For this review, take the finished solid that the model builds, in its own axes (mm). A direction names the side the tool comes from. Coordinates: 2 decimals unless noted, no trailing zeros. Loops run counter-clockwise (first coordinate to the right, second up) from the corner with the lowest first, then second, coordinate; pieces in that order, holes last. Notation, with made-up numbers: M 72.5,68.5 L 103.5,68.5 A12 cw 103.5,73.5 Z; hole C 65,-14.5 d6. An arc over 180 degrees is marked long. Answer as a JSON object with one key per item and string values. Group by question number.
Item 1: Add section A-A (x = -9.5). State the section outline as (y, z) points, then the cut area to 3 significant figures.
Item 2: Insertion check: pin 1 (1 mm diameter, centred on x = 9, z = -35, fed in from +Y); pin 2 (3 mm diameter, centred on x = 39, z = -39, fed in from -Y); pin 3 (1 mm diameter, centred on x = 6, y = 0.5, fed in from -Z); pin 4 (1.6 mm diameter, centred on x = 43.5, y = 3, fed in from +Z). Each pin has a flat end and moves straight along its axis. Give the tip position at first contact, or say it passes through.
Item 3: Tool access review of faces 4 (the face through (42, 3, -32.785)), 5 (the face through (-42, 3, 32.785)), 6 (the face through (33.607, 1.014, -44.132)), 7 (the face through (0, 1, 40.021)): name each direction out of +Z, -Z, +X, -X, +Y, -Y from which nothing blocks a thin tool from reaching the whole face with its end or side.
Item 4: Wall thickness on L1, parallel to X at y = 1, z = -39; L2, parallel to Z at x = 11, y = 0.2; L3, parallel to X at y = 3.45, z = -20: over which ranges is each line inside the solid? List them lowest first. Write a range as from..to.
Item 5: Mouldability with a two-part tool opening along Z and no side actions: class faces 1 (the face through (42, 3, 32.785)), 2 (the face through (37.418, 0.986, -41.063)), 3 (the face through (-42, 3, -32.785)) as +Z half, -Z half, draft (parallel to the pull), parting line (faces both ways), or undercut.
Item 6: Add section D-D (z = 39). State the section outline as (x, y) points.
Item 7: Add section C-C (y = 2.95). State the section outline as (x, z) points, then the cut area to 3 significant figures.
Item 8: Add section B-B (z = -24). State the section outline as (x, y) points.
from build123d import *

# Parameters (mm, degrees)
SKETCH_1_W          = 90.03018306390481
SKETCH_1_H          = 89.97022234109225
SKETCH_1_R          = 2.599999999999996
SKETCH_1_W_2        = 65.97077516555349
SKETCH_1_H_2        = 66.02977765890743
EXTRUDE_1_DEPTH     = 2
CUT_EXTRUDE_1_DEPTH = 64.67117630966501
CUT_EXTRUDE_2_DEPTH = 64.67117630966501
EXTRUDE_START       = 2
EXTRUDE_2_DEPTH     = 2
FILLET_1_R          = 1


with BuildPart() as part:
    # 草图1 → 凸台-拉伸1 (new body)
    with BuildSketch(Plane(origin=(0, 0, 0), x_dir=(1, 0, 0), z_dir=(0, 1, 0))):
        Rectangle(SKETCH_1_W, SKETCH_1_H)
        with Locations(Location((39.00000000000001, 38.99999999999999, 0), (0, 0, 270))):
            Circle(SKETCH_1_R, mode=Mode.SUBTRACT)
        with Locations(Location((39.000000000000014, -39.00000000000001, 0), (0, 0, 270))):
            Circle(SKETCH_1_R, mode=Mode.SUBTRACT)
        with Locations(Location((-38.99999999999998, -39.00000000000001, 0), (0, 0, 270))):
            Circle(SKETCH_1_R, mode=Mode.SUBTRACT)
        with Locations(Location((-38.99999999999999, 38.99999999999999, 0), (0, 0, 270))):
            Circle(SKETCH_1_R, mode=Mode.SUBTRACT)
        Rectangle(SKETCH_1_W_2, SKETCH_1_H_2, mode=Mode.SUBTRACT)
    extrude(amount=EXTRUDE_1_DEPTH)

    # 草图3 → 切除-拉伸1 (cut, through all)
    with BuildSketch(Plane(origin=(0, 2, 0), x_dir=(1, 0, 0), z_dir=(0, 1, 0))):
        with BuildLine():
            Line((35.16632906527342, 44.985111170546105), (-35.16632906527342, 44.985111170546126))
            ThreePointArc((-35.16632906527342, 44.98511117054611), (-33.623759393307296, 44.150934913211564), (-33.00868514907322, 42.50866365204603))
            ThreePointArc((-33.00868514907322, 42.50866365204603), (-32.2698933068484, 40.74672362699537), (-30.502504505895168, 40.02106333162392))
            Line((-30.502504505895168, 40.02106333162392), (30.502504505895196, 40.0210633316239))
            ThreePointArc((30.502504505895196, 40.0210633316239), (32.269893306848424, 40.74672362699535), (33.00868514907325, 42.50866365204601))
            ThreePointArc((33.00868514907325, 42.50866365204601), (33.62375939330732, 44.150934913211536), (35.16632906527342, 44.98511117054609))
        make_face()
        with BuildLine():
            Line((30.502504505895207, -40.0210633316239), (-30.502504505895114, -40.02106333162392))
            ThreePointArc((-30.502504505895114, -40.02106333162392), (-32.269893306848346, -40.74672362699537), (-33.008685149073166, -42.50866365204603))
            ThreePointArc((-33.008685149073166, -42.50866365204603), (-33.62375939330724, -44.150934913211564), (-35.166329065273366, -44.98511117054611))
            Line((-35.166329065273366, -44.985111170546126), (35.16632906527344, -44.985111170546105))
            ThreePointArc((35.16632906527343, -44.98511117054609), (33.623759393307324, -44.150934913211536), (33.00868514907326, -42.50866365204601))
            ThreePointArc((33.00868514907326, -42.50866365204601), (32.26989330684843, -40.74672362699535), (30.502504505895203, -40.0210633316239))
        make_face()
    extrude(amount=-CUT_EXTRUDE_1_DEPTH, mode=Mode.SUBTRACT)

    # 草图4 → 切除-拉伸2 (cut, through all)
    with BuildSketch(Plane(origin=(0, 2, 0), x_dir=(1, 0, 0), z_dir=(0, 1, 0))):
        with BuildLine():
            Line((-32.985387582776745, -33.01488882945372), (-32.985387582776724, 33.01488882945372))
            ThreePointArc((-32.985387582776724, 33.01488882945372), (-37.9510386162303, 30.950835913733954), (-40.0150915319524, 25.985184880281345))
            Line((-40.01509153195237, 25.985184880281345), (-40.01509153195237, 25.95025335742635))
            Line((-40.01509153195237, 25.95025335742635), (-40.0150915319524, -25.95025335742637))
            Line((-40.0150915319524, -25.95025335742637), (-40.0150915319524, -25.985184880281345))
            ThreePointArc((-40.015091531952386, -25.985184880281345), (-37.95103861623032, -30.950835913733957), (-32.985387582776745, -33.01488882945372))
        make_face()
        with BuildLine():
            Line((40.01509153195237, 25.950253357426362), (40.01509153195237, 25.985184880281345))
            ThreePointArc((40.0150915319524, 25.985184880281345), (37.9510386162303, 30.95083591373395), (32.985387582776724, 33.01488882945372))
            Line((32.985387582776724, 33.01488882945372), (32.985387582776745, -33.01488882945372))
            ThreePointArc((32.985387582776745, -33.01488882945372), (37.95103861623032, -30.950835913733957), (40.0150915319524, -25.985184880281345))
            Line((40.0150915319524, -25.985184880281345), (40.0150915319524, -25.950253357426362))
            Line((40.0150915319524, -25.950253357426362), (40.01509153195237, 25.950253357426362))
        make_face()
    extrude(amount=-CUT_EXTRUDE_2_DEPTH, mode=Mode.SUBTRACT)

    # 草图5 → 凸台-拉伸2 (add)
    with BuildSketch(Plane(origin=(0, 2, 0), x_dir=(1, 0, 0), z_dir=(0, 1, 0)).offset(EXTRUDE_START)):
        with BuildLine():
            Line((45.015091531952415, -32.78514802541212), (45.015091531952415, 32.78514802541212))
            Line((45.015091531952415, 32.78514802541212), (34.75273808271875, 32.78514802541212))
            ThreePointArc((34.75273808271875, 32.78514802541213), (38.54114967835172, 30.28072702943986), (40.01509153195237, 25.985184880281345))
            Line((40.01509153195237, 25.985184880281345), (40.0150915319524, -25.985184880281345))
            ThreePointArc((40.0150915319524, -25.985184880281345), (38.54114967835175, -30.280727029439863), (34.75273808271877, -32.78514802541212))
            Line((34.75273808271877, -32.78514802541212), (45.015091531952415, -32.78514802541212))
        make_face()
        with BuildLine():
            Line((-45.01509153195241, 32.78514802541209), (-45.01509153195241, -32.78514802541212))
            Line((-45.0150915319524, -32.78514802541212), (-34.75273808271877, -32.78514802541212))
            ThreePointArc((-34.75273808271877, -32.78514802541212), (-38.54114967835175, -30.280727029439863), (-40.0150915319524, -25.985184880281345))
            Line((-40.0150915319524, -25.985184880281345), (-40.01509153195237, 25.985184880281345))
            ThreePointArc((-40.01509153195237, 25.985184880281345), (-38.54114967835173, 30.280727029439863), (-34.75273808271875, 32.78514802541213))
            Line((-34.75273808271875, 32.78514802541212), (-45.01509153195241, 32.78514802541209))
        make_face()
    extrude(amount=-EXTRUDE_2_DEPTH)

    # 圆角1
    fillet_1_edges = [part.edges().sort_by_distance(p)[0] for p in [
        (34.75273808271877, 3, 32.78514802541213),
        (34.75273808271875, 3, -32.78514802541213),
        (-34.75273808271875, 3, -32.78514802541213),
        (-34.75273808271877, 3, 32.78514802541212),
    ]]
    fillet(fillet_1_edges, radius=FILLET_1_R)


solid = part.part
From the geometry:
{
 "1": {"outline": "M 0,-40.02 L 2,-40.02 L 2,-33.01 L 0,-33.01 Z; M 0,33.01 L 2,33.01 L 2,40.02 L 0,40.02 Z", "area": "28.0 mm²"},
 "2": {"pin 1": "stops at y = 2", "pin 2": "passes through", "pin 3": "stops at z = -40.02", "pin 4": "stops at z = 32.79"},
 "3": {"face 4": "-Z, +X, -X, +Y", "face 5": "+Z, +X, -X, +Y", "face 6": "-Z, +Y, -Y", "face 7": "+Z, +Y, -Y"},
 "4": {"L1": "x = -45.02..-41.6, -36.4..36.4, 41.6..45.02", "L2": "z = -40.02..-33.01, 33.01..40.02", "L3": "x = -45.02..-40.02, 40.02..45.02"},
 "5": {"face 1": "+Z half", "face 2": "undercut", "face 3": "-Z half"},
 "6": {"outline": "M -45.02,0 L -41.6,0 L -41.6,2 L -45.02,2 Z; M -36.4,0 L 36.4,0 L 36.4,2 L -36.4,2 Z; M 41.6,0 L 45.02,0 L 45.02,2 L 41.6,2 Z"},
 "7": {"outline": "M -45.02,-32.79 L -38.53,-32.79 A1 ccw -37.84,-31.06 A7.05 cw -40.02,-25.99 L -40.02,25.99 A7.05 cw -37.84,31.06 A1 ccw -38.53,32.79 L -45.02,32.79 Z; M 37.84,-31.06 A1 ccw 38.53,-32.79 L 45.02,-32.79 L 45.02,32.79 L 38.53,32.79 A1 ccw 37.84,31.06 A7.05 cw 40.02,25.99 L 40.02,-25.99 A7.05 cw Z", "area": "685 mm²"},
 "8": {"outline": "M -45.02,0 L -40.02,0 L -40.02,4 L -45.02,4 Z; M 40.02,0 L 45.02,0 L 45.02,4 L 40.02,4 Z"}
}
